```python
from build123d import *

# Parameters (mm, degrees)
EXTRUDE_1_DEPTH     = 4
SKETCH_2_W          = 10
SKETCH_2_H          = 210
SKETCH_2_W_2        = 210
SKETCH_2_H_2        = 10
CUT_EXTRUDE_1_DEPTH = 2
SKETCH_3_W          = 210
SKETCH_3_H          = 10
SKETCH_3_W_2        = 10
SKETCH_3_H_2        = 210
CUT_EXTRUDE_2_DEPTH = 2
SKETCH_4_R          = 2.5
CUT_EXTRUDE_3_DEPTH = 326.293713434
SKETCH_5_W          = 190
SKETCH_5_H          = 40
CUT_EXTRUDE_4_DEPTH = 326.293713434


with BuildPart() as part:
    # 草图1 → 凸台-拉伸1 (new body)
    with BuildSketch(Plane.XY):
        Polygon((10, 0), (10, 10), (0, 10), (0, 220), (10, 220), (10, 230), (220, 230), (220, 220), (230, 220), (230, 10), (220, 10), (220, 0), align=None)
    extrude(amount=EXTRUDE_1_DEPTH)

    # 草图2 → 切除-拉伸1 (cut)
    with BuildSketch(Plane.XY.offset(4)):
        with Locations((225, 115)):
            Rectangle(SKETCH_2_W, SKETCH_2_H)
        with Locations((115, 5)):
            Rectangle(SKETCH_2_W_2, SKETCH_2_H_2)
    extrude(amount=-CUT_EXTRUDE_1_DEPTH, mode=Mode.SUBTRACT)

    # 草图3 → 切除-拉伸2 (cut)
    with BuildSketch(Plane(origin=(0, 0, 0), x_dir=(-1, 0, 0), z_dir=(0, 0, -1))):
        with Locations((-115, 225)):
            Rectangle(SKETCH_3_W, SKETCH_3_H)
        with Locations((-5, 115)):
            Rectangle(SKETCH_3_W_2, SKETCH_3_H_2)
    extrude(amount=-CUT_EXTRUDE_2_DEPTH, mode=Mode.SUBTRACT)

    # 草图4 → 切除-拉伸3 (cut, through all)
    with BuildSketch(Plane.XY.offset(4)):
        with Locations((5, 80)):
            Circle(SKETCH_4_R)
        with Locations((5, 90)):
            Circle(SKETCH_4_R)
        with Locations(Location((5, 150, 0), (0, 0, 180))):
            Circle(SKETCH_4_R)
        with Locations(Location((5, 140, 0), (0, 0, 180))):
            Circle(SKETCH_4_R)
        with Locations((225, 80)):
            Circle(SKETCH_4_R)
        with Locations((225, 90)):
            Circle(SKETCH_4_R)
        with Locations((225, 140)):
            Circle(SKETCH_4_R)
        with Locations((225, 150)):
            Circle(SKETCH_4_R)
        with Locations((80, 5)):
            Circle(SKETCH_4_R)
        with Locations((90, 5)):
            Circle(SKETCH_4_R)
        with Locations((140, 5)):
            Circle(SKETCH_4_R)
        with Locations((150, 5)):
            Circle(SKETCH_4_R)
        with Locations((150, 225)):
            Circle(SKETCH_4_R)
        with Locations((140, 225)):
            Circle(SKETCH_4_R)
        with Locations(Location((90, 225, 0), (0, 0, 180))):
            Circle(SKETCH_4_R)
        with Locations(Location((80, 225, 0), (0, 0, 180))):
            Circle(SKETCH_4_R)
    extrude(amount=-CUT_EXTRUDE_3_DEPTH, mode=Mode.SUBTRACT)

    # 草图5 → 切除-拉伸4 (cut, through all)
    with BuildSketch(Plane.XY.offset(4)):
        with Locations((115, 40)):
            Rectangle(SKETCH_5_W, SKETCH_5_H)
        with Locations((115, 90)):
            Rectangle(SKETCH_5_W, SKETCH_5_H)
        with Locations((115, 140)):
            Rectangle(SKETCH_5_W, SKETCH_5_H)
        with Locations((115, 190)):
            Rectangle(SKETCH_5_W, SKETCH_5_H)
    extrude(amount=-CUT_EXTRUDE_4_DEPTH, mode=Mode.SUBTRACT)


solid = part.part
```
CAD build for the part. Positions are in the model's coordinates, mm. A direction names the side the tool comes from. Round coordinates to 2 decimals unless told otherwise and drop trailing zeros. Order: outer loops, then holes, each group sorted by start corner. A loop starts at its lowest first (then second) coordinate and runs counter-clockwise, first axis right, second up.
Item 1: Probe line 1 along Y through (x, z) = (182, 1); line 2 along Y through (x, z) = (113.5, 3.4); line 3 along Y through (x, z) = (150, 3.05). List the from-to ranges inside material, lowest first.
Item 2: Mould opens along Y. For faces 6 (the face through (151.34, 227.11, 3.01)), 7 (the face through (122, 112, 0)), 8 (the face through (5.33, 137.52, 3.01)) say: pulls with the +Y half, pulls with the -Y half, needs draft (parallel to the pull), parting line crosses it, or undercut.
Item 3: Saw through at A-A on y = 202.5. Write the cut outline in (x, z).
Item 4: Saw through at D-D on y = 164. Write the cut outline in (x, z).
Item 5: Tool access for faces 1 (the face through (5, 116, 2)), 2 (the face through (116, 225, 2)), 3 (the face through (227.31, 79.04, 1.01)), 4 (the face through (225, 116, 2)), 5 (the face through (114, 5, 2)): list every direction of +Z, -Z, +X, -X, +Y, -Y with a clear straight run to the whole face (end or side of a thin tool).
Item 6: Saw through at B-B on z = 3. State how many separate pieces and enclosed holes the cut face has, then the cut area to 3 significant figures.
Item 7: Saw through at C-C on x = 47. Write the cut outline in (y, z).
Item 8: Pin check, flat tips, straight feed: pin 1 (5 mm diameter, centred on x = 5, y = 149.5, fed in from -Z); pin 2 (1.6 mm diameter, centred on x = 226.5, z = 1.5, fed in from -Y); pin 3 (11 mm diameter, centred on x = 128, y = 5, fed in from +Z); pin 4 (2 mm diameter, centred on y = 104.5, z = 3.5, fed in from +X). Stop position of each tip, or through.
Reported:
1. line 1: y = 0 to 20, 60 to 70, 110 to 120, 160 to 170, 210 to 220
1. line 2: y = 10 to 20, 60 to 70, 110 to 120, 160 to 170, 210 to 230
1. line 3: y = 10 to 20, 60 to 70, 110 to 120, 160 to 170, 210 to 222.5, 227.5 to 230
2. face 6: undercut
2. face 7: needs draft
2. face 8: undercut
3. outline: (0, 2) - (10, 2) - (10, 0) - (20, 0) - (20, 4) - (0, 4) - close; (210, 0) - (230, 0) - (230, 2) - (220, 2) - (220, 4) - (210, 4) - close
4. outline: (0, 2) - (10, 2) - (10, 0) - (230, 0) - (230, 2) - (220, 2) - (220, 4) - (0, 4) - close
5. face 1: -Z, -X, +Y, -Y
5. face 2: -Z, +X, -X, +Y
5. face 3: +Z, -Z
5. face 4: +Z, +X, +Y, -Y
5. face 5: +Z, +X, -X, -Y
6. separate pieces: 1
6. enclosed holes: 12
6. area: 17,700 mm2
7. outline: (0, 0) - (20, 0) - (20, 4) - (10, 4) - (10, 2) - (0, 2) - close; (60, 0) - (70, 0) - (70, 4) - (60, 4) - close; (110, 0) - (120, 0) - (120, 4) - (110, 4) - close; (160, 0) - (170, 0) - (170, 4) - (160, 4) - close; (210, 0) - (220, 0) - (220, 2) - (230, 2) - (230, 4) - (210, 4) - close
8. pin 1: stops at z = 2
8. pin 2: stops at y = 10
8. pin 3: stops at z = 4
8. pin 4: stops at x = 220
